```python
from build123d import *

# Parameters (mm, degrees)
F0_R     = 11.049
F1_DEPTH = 6.35


with BuildPart() as f1:
    # F0 (on Top) → F1 (new body)
    with BuildSketch(Plane.XY):
        with BuildLine():
            ThreePointArc((13.629375726, -17.2792417221), (17.7003329036, -7.4217648034), (27.5405927913, -3.309365396))
            ThreePointArc((27.5405927913, -3.309365396), (15.086449318, 7.051761798), (11.7361280198, 22.9021243674))
            ThreePointArc((11.7361280198, 22.9021243674), (6.6819898762, 18.2116703951), (0, 16.51))
            ThreePointArc((0, 16.51), (-6.6763170276, 18.2085823579), (-11.7291158994, 22.891275455))
            ThreePointArc((-11.7291158994, 22.891275455), (-15.0856557039, 7.0272020842), (-27.5610287338, -3.3313813683))
            ThreePointArc((-27.5610287338, -3.3313813683), (-17.6827470006, -7.4230996351), (-13.5910287338, -17.3013813683))
            ThreePointArc((-13.5910287338, -17.3013813683), (0.0166082519, -14.1363774408), (13.629375726, -17.2792417221))
        make_face()
        with BuildLine():
            ThreePointArc((13.97, 0), (-9.8782817332, -9.8782817332), (0, 13.97))
            ThreePointArc((0, 13.97), (9.8782817332, 9.8782817332), (13.97, 0))
        make_face(mode=Mode.SUBTRACT)
        with BuildLine():
            ThreePointArc((13.97, 0), (9.8782817332, 9.8782817332), (0, 13.97))
            ThreePointArc((0, 13.97), (-9.8782817332, -9.8782817332), (13.97, 0))
        make_face()
        with BuildLine():
            ThreePointArc((11.049, 0), (-7.8128228253, -7.8128228253), (0, 11.049))
            ThreePointArc((0, 11.049), (7.8128228253, 7.8128228253), (11.049, 0))
        make_face(mode=Mode.SUBTRACT)
        with BuildLine():
            ThreePointArc((13.97, 30.48), (9.8782817686, 40.3582816978), (1.001e-07, 44.45))
            ThreePointArc((1.001e-07, 44.45), (-9.8782816978, 40.3582817686), (-13.97, 30.48))
            ThreePointArc((-13.97, 30.48), (-12.5435043089, 26.7760126955), (-11.7291158994, 22.891275455))
            ThreePointArc((-11.7291158994, 22.891275455), (-6.6763170276, 18.2085823579), (0, 16.51))
            ThreePointArc((0, 16.51), (6.6819898762, 18.2116703951), (11.7361280198, 22.9021243674))
            ThreePointArc((11.7361280198, 22.9021243674), (12.5479892343, 26.7809947751), (13.97, 30.48))
        make_face()
        with BuildLine():
            ThreePointArc((11.049, 30.48), (7.8128228253, 22.6671771747), (0, 19.431))
            ThreePointArc((0, 19.431), (-7.8128228253, 38.2928228253), (11.049, 30.48))
        make_face(mode=Mode.SUBTRACT)
        with BuildLine():
            ThreePointArc((-27.5610287338, -3.3313813683), (-36.9681276962, -6.9733908033), (-41.4703242711, -16.0004595199))
            ThreePointArc((-41.4703242711, -16.0004595199), (-37.6469546626, -23.6328014554), (-32.4351043479, -30.3935273692))
            ThreePointArc((-32.4351043479, -30.3935273692), (-19.5901422188, -28.7742131096), (-13.5910287338, -17.3013813683))
            ThreePointArc((-13.5910287338, -17.3013813683), (-17.6827470006, -7.4230996351), (-27.5610287338, -3.3313813683))
        make_face()
        with Locations((-27.5610287338, -17.3013813683)):
            Circle(F0_R, mode=Mode.SUBTRACT)
        with BuildLine():
            ThreePointArc((32.4464596099, -30.3814048191), (37.6753336679, -23.5875334236), (41.5027242234, -15.9162301452))
            ThreePointArc((41.5027242234, -15.9162301452), (36.9616008144, -6.9105561066), (27.5405927913, -3.309365396))
            ThreePointArc((27.5405927913, -3.309365396), (17.7003329036, -7.4217648034), (13.629375726, -17.2792417221))
            ThreePointArc((13.629375726, -17.2792417221), (19.6166713552, -28.7438538363), (32.4464596099, -30.3814048191))
        make_face()
        with Locations((27.599375726, -17.2792417221)):
            Circle(F0_R, mode=Mode.SUBTRACT)
        with BuildLine():
            ThreePointArc((41.569375726, -17.2792417221), (41.552702901, -16.5969216026), (41.5027242234, -15.9162301452))
            ThreePointArc((41.5027242234, -15.9162301452), (37.6753336679, -23.5875334236), (32.4464596099, -30.3814048191))
            ThreePointArc((32.4464596099, -30.3814048191), (39.0639878402, -25.2619460928), (41.569375726, -17.2792417221))
        make_face()
        with BuildLine():
            ThreePointArc((-32.4351043479, -30.3935273692), (-37.6469546626, -23.6328014554), (-41.4703242711, -16.0004595199))
            ThreePointArc((-41.4703242711, -16.0004595199), (-39.3929287706, -24.7288332543), (-32.4351043479, -30.3935273692))
        make_face()
    extrude(amount=F1_DEPTH)


solid = f1.part
```
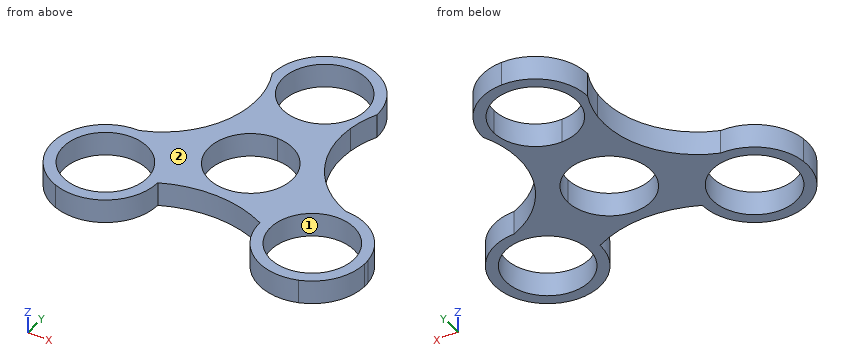
The model under review builds one solid part; all positions refer to its coordinate system, in mm. Face numbers are marked on the shaded views. Round coordinates to 2 decimals unless told otherwise and drop trailing zeros. Order: outer loops, then holes, each group sorted by start corner. A loop starts at its lowest first (then second) coordinate and runs counter-clockwise, first axis right, second up. Notation, with made-up numbers: (55, -20.75) -> (76, -20.75) arc R15 ccw to (76, 3.25) -> close; hole circle Ø5 at (-26.75, 56.5). An arc over 180 degrees is marked (long way). Use a Markdown table: item, result.
Q1. We need section D-D on x = -21. Write out the cut boundary in (y, z).
Values:
| item | result |
|---|---|
| outline | (-29.63, 0) -> (-26.19, 0) -> (-26.19, 6.35) -> (-29.63, 6.35) -> close; (-8.41, 0) -> (0.35, 0) -> (0.35, 6.35) -> (-8.41, 6.35) -> close |
Q2. Mouldability with a two-part tool opening along X and no side actions: class the marked faces 1 and 2 as +X half, -X half, draft (parallel to the pull), parting line (faces both ways), or undercut.
Values:
| item | result |
|---|---|
| face 1 | undercut |
| face 2 | draft |
Q3. We need section A-A on z = 3.25. Write out the cut boundary in (x, y), then the cut area to 3 significant figures.
Values:
| item | result |
|---|---|
| outline | (-27.56, -3.33) arc R13.97 ccw (long way) to (-13.59, -17.3) arc R30.94 cw to (13.63, -17.28) arc R13.97 ccw (long way) to (27.54, -3.31) arc R24.69 cw to (13.97, 30.48) arc R13.97 ccw to (-13.97, 30.48) arc R24.68 cw to start; hole circle Ø22.1 at (-27.56, -17.3); hole circle Ø22.1 at (0, 0); hole circle Ø22.1 at (0, 30.48); hole circle Ø22.1 at (27.6, -17.28) |
| area | 1,400 mm^2 |
Q4. Clearance check with flat-ended pins moving along their axes: P1, Ø17.5, axis at x = 0, y = 0, coming from the -Z side; P2, Ø3, axis at x = 17.5, z = 4.5, coming from the +Y side. State where each tip first meets the part, or that it passes through.
Values:
| item | result |
|---|---|
| P1 | passes through |
| P2 | stops at y = 5.65 |
Q5. We need section C-C on y = -13. Write out the cut boundary in (x, z).
Values:
| item | result |
|---|---|
| outline | (-40.85, 0) -> (-37.74, 0) -> (-37.74, 6.35) -> (-40.85, 6.35) -> close; (-17.38, 0) -> (17.41, 0) -> (17.41, 6.35) -> (-17.38, 6.35) -> close; (37.79, 0) -> (40.9, 0) -> (40.9, 6.35) -> (37.79, 6.35) -> close |
Q6. We need section B-B on x = -6. Write out the cut boundary in (y, z), then the cut area to 3 significant figures.
Values:
| item | result |
|---|---|
| outline | (-14.73, 0) -> (-9.28, 0) -> (-9.28, 6.35) -> (-14.73, 6.35) -> close; (9.28, 0) -> (21.2, 0) -> (21.2, 6.35) -> (9.28, 6.35) -> close; (39.76, 0) -> (43.1, 0) -> (43.1, 6.35) -> (39.76, 6.35) -> close |
| area | 132 mm^2 |
Q7. For line 1 (Y direction, x = -1.5, z = 1); line 2 (Y direction, x = 10, z = 5.75); line 3 (Y direction, x = -29.5, z = 4.5), list the stretches that pass through material, from the lowest coordinate up.
Values:
| item | result |
|---|---|
| line 1 | y = -14.17 to -10.95, 10.95 to 19.53, 41.43 to 44.37 |
| line 2 | y = -15.78 to -4.7, 4.7 to 25.78, 35.18 to 40.24 |
| line 3 | y = -31.14 to -28.18, -6.42 to -3.47 |
